Model file for the job. Use its own axes, mm. A direction names the side the tool comes from. Round coordinates to 2 decimals unless told otherwise and drop trailing zeros. Loops run counter-clockwise (first coordinate to the right, second up) from the corner with the lowest first, then second, coordinate; pieces in that order, holes last. Notation, with made-up numbers: (41, -5) -> (75, -5) arc R13 cw to (75, 17) -> close; hole circle Ø1 at (-29, -2). An arc over 180 degrees is marked (long way). Use a Markdown table: item, result. Add a question column.
```python
from build123d import *

# Parameters (mm, degrees)
SKETCH1_W           = 45
SKETCH1_H           = 42
BOSS_EXTRUDE1_DEPTH = 4
SKETCH2_R           = 1.75
CUT_EXTRUDE1_DEPTH  = 32.036269106
SKETCH3_R           = 1.75
CUT_EXTRUDE2_DEPTH  = 32.036269106
CUT_EXTRUDE4_DEPTH  = 2


with BuildPart() as part:
    # Sketch1 → Boss-Extrude1 (new body)
    with BuildSketch(Plane.XY):
        Rectangle(SKETCH1_W, SKETCH1_H)
    extrude(amount=BOSS_EXTRUDE1_DEPTH)

    # Sketch2 → Cut-Extrude1 (cut, through all)
    with BuildSketch(Plane.XY.offset(4)):
        with Locations((-17.5, 16)):
            Circle(SKETCH2_R)
        with Locations((-2.5, 16)):
            Circle(SKETCH2_R)
        with Locations(Location((-2.5, -16, 0), (0, 0, 180))):
            Circle(SKETCH2_R)
        with Locations(Location((-17.5, -16, 0), (0, 0, 180))):
            Circle(SKETCH2_R)
    extrude(amount=-CUT_EXTRUDE1_DEPTH, mode=Mode.SUBTRACT)

    # Sketch3 → Cut-Extrude2 (cut, through all)
    with BuildSketch(Plane.XY.offset(4)):
        with Locations((12.5, 16)):
            Circle(SKETCH3_R)
        with Locations(Location((12.5, -16, 0), (0, 0, 180))):
            Circle(SKETCH3_R)
    extrude(amount=-CUT_EXTRUDE2_DEPTH, mode=Mode.SUBTRACT)

    # Sketch5 → Cut-Extrude4 (cut)
    with BuildSketch(Plane(origin=(0, 0, 0), x_dir=(-1, 0, 0), z_dir=(0, 0, -1))):
        Polygon((-9.209103466, -16), (-10.854551733, -13.15), (-14.145448267, -13.15), (-15.790896534, -16), (-14.145448267, -18.85), (-10.854551733, -18.85), align=None)
        Polygon((-10.854551733, 18.85), (-9.209103466, 16), (-10.854551733, 13.15), (-14.145448267, 13.15), (-15.790896534, 16), (-14.145448267, 18.85), align=None)
    extrude(amount=-CUT_EXTRUDE4_DEPTH, mode=Mode.SUBTRACT)


solid = part.part
```
1) Cut at B-B on z = 3. Write the cut outline in (x, y).
2) Tool access for faces 1 (the face through (12.728, -17.735, 3.014)), 2 (the face through (14.96, 14.56, 0.99)): list every direction of +Z, -Z, +X, -X, +Y, -Y with a clear straight run to the whole face (end or side of a thin tool).
3) Cut at C-C on y = -16.5. Write the cut outline in (x, z), and give its area (3 significant figures).
4) Cut at D-D on x = -17. Write the cut outline in (y, z).
5) Pull direction X, two halves, no side cores. Call faces 3 (the face through (-22.5, 0, 2)), 4 (the face through (0, -21, 2)), 5 (the face through (-18.79, 17.18, 2.03)): +X half, -X half, draft (parallel to the pull), parting line (faces both ways), or undercut.
6) Cut at A-A on x = -2.5. Write the cut outline in (y, z).
7) Wall check: probe 1 along X at (y, z) = (-16, 0.4); probe 2 along Y at (x, z) = (12.5, 2.9); probe 3 along X at (y, z) = (-16, 3.5). Give the ranges that are in metal, low to high. Write a range as from..to.
Established:
| question | item | result |
|---|---|---|
| 1 | outline | (-22.5, -21) -> (22.5, -21) -> (22.5, 21) -> (-22.5, 21) -> close; hole circle Ø3.5 at (-17.5, -16); hole circle Ø3.5 at (-17.5, 16); hole circle Ø3.5 at (-2.5, -16); hole circle Ø3.5 at (-2.5, 16); hole circle Ø3.5 at (12.5, -16); hole circle Ø3.5 at (12.5, 16) |
| 2 | face 1 | +Z, -Z |
| 2 | face 2 | -Z |
| 3 | outline | (-22.5, 0) -> (-19.18, 0) -> (-19.18, 4) -> (-22.5, 4) -> close; (-15.82, 0) -> (-4.18, 0) -> (-4.18, 4) -> (-15.82, 4) -> close; (-0.82, 0) -> (9.5, 0) -> (9.5, 2) -> (10.82, 2) -> (10.82, 4) -> (-0.82, 4) -> close; (14.18, 2) -> (15.5, 2) -> (15.5, 0) -> (22.5, 0) -> (22.5, 4) -> (14.18, 4) -> close |
| 3 | area | 134 mm^2 |
| 4 | outline | (-21, 0) -> (-17.68, 0) -> (-17.68, 4) -> (-21, 4) -> close; (-14.32, 0) -> (14.32, 0) -> (14.32, 4) -> (-14.32, 4) -> close; (17.68, 0) -> (21, 0) -> (21, 4) -> (17.68, 4) -> close |
| 5 | face 3 | -X half |
| 5 | face 4 | draft |
| 5 | face 5 | undercut |
| 6 | outline | (-21, 0) -> (-17.75, 0) -> (-17.75, 4) -> (-21, 4) -> close; (-14.25, 0) -> (14.25, 0) -> (14.25, 4) -> (-14.25, 4) -> close; (17.75, 0) -> (21, 0) -> (21, 4) -> (17.75, 4) -> close |
| 7 | probe 1 | x = -22.5..-19.25, -15.75..-4.25, -0.75..9.21, 15.79..22.5 |
| 7 | probe 2 | y = -21..-17.75, -14.25..14.25, 17.75..21 |
| 7 | probe 3 | x = -22.5..-19.25, -15.75..-4.25, -0.75..10.75, 14.25..22.5 |
